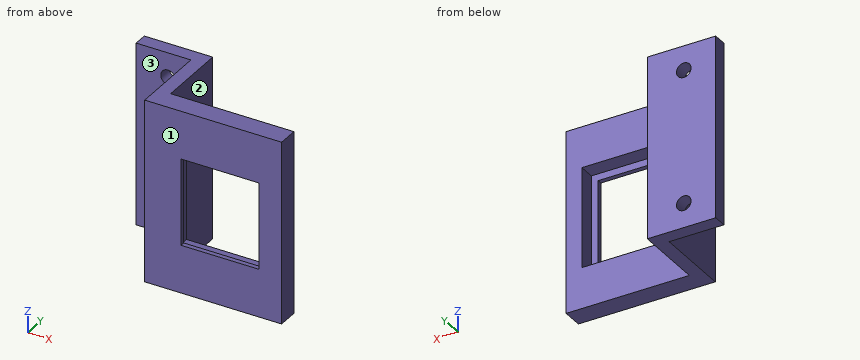
from build123d import *

# Parameters (mm, degrees)
BOSS_EXTRUDE1_DEPTH = 40
SKETCH2_W           = 20.1
SKETCH2_H           = 22
CUT_EXTRUDE1_DEPTH  = 3.5
SKETCH3_W           = 17.1
SKETCH3_H           = 19
CUT_EXTRUDE2_DEPTH  = 54.488316481
SKETCH4_R           = 1.6
CUT_EXTRUDE3_DEPTH  = 54.851648071


with BuildPart() as part:
    # Sketch1 → Boss-Extrude1 (new body)
    with BuildSketch(Plane.XY):
        Polygon((0, 0), (0, 17), (-12, 17), (-12, 20), (3, 20), (3, 4.5), (30, 4.5), (30, 0), align=None)
    extrude(amount=-BOSS_EXTRUDE1_DEPTH)

    # Sketch2 → Cut-Extrude1 (cut)
    with BuildSketch(Plane(origin=(0, 4.5, 0), x_dir=(1, 0, 0), z_dir=(0, 1, 0))):
        with Locations((16.5, 20)):
            Rectangle(SKETCH2_W, SKETCH2_H)
    extrude(amount=-CUT_EXTRUDE1_DEPTH, mode=Mode.SUBTRACT)

    # Sketch3 → Cut-Extrude2 (cut, through all)
    with BuildSketch(Plane(origin=(0, 1, 0), x_dir=(1, 0, 0), z_dir=(0, 1, 0))):
        with Locations((16.5, 20)):
            Rectangle(SKETCH3_W, SKETCH3_H)
    extrude(amount=-CUT_EXTRUDE2_DEPTH, mode=Mode.SUBTRACT)

    # Sketch4 → Cut-Extrude3 (cut, through all)
    with BuildSketch(Plane(origin=(0, 20, 0), x_dir=(1, 0, 0), z_dir=(0, 1, 0))):
        with Locations(Location((-5, 34.63, 0), (0, 0, 270))):
            Circle(SKETCH4_R)
        with Locations(Location((-5, 5.366, 0), (0, 0, 270))):
            Circle(SKETCH4_R)
    extrude(amount=-CUT_EXTRUDE3_DEPTH, mode=Mode.SUBTRACT)


solid = part.part
For this review, take the finished solid that the model builds, in its own axes (mm). Face numbers are marked on the shaded views. A direction names the side the tool comes from. Round coordinates to 2 decimals unless told otherwise and drop trailing zeros. Order: outer loops, then holes, each group sorted by start corner. A loop starts at its lowest first (then second) coordinate and runs counter-clockwise, first axis right, second up. Notation, with made-up numbers: M 15.25,82 L 60.25,82 A18 ccw 60.25,86 Z; hole C 55,-2.75 d3. An arc over 180 degrees is marked long. Use a Markdown table: item, result. Add a question column.
Item 1: Insertion check: pin 1 (0.5 mm diameter, centred on y = 0.5, z = -23, fed in from -X); pin 2 (1.5 mm diameter, centred on x = 10, z = -15, fed in from -Y); pin 3 (1.5 mm diameter, centred on y = 8.5, z = -22.5, fed in from +X); pin 4 (16 mm diameter, centred on x = 19.5, z = -15.5, fed in from +Y). Each pin has a flat end and moves straight along its axis. Give the tip position at first contact, or say it passes through.
Item 2: Add section D-D, the plane z = -34.63. Give the boundary of the cut face in (x, y), then the cut area to 3 significant figures.
Item 3: Add section A-A, the plane x = 9. Give the boundary of the cut face in (y, z).
Item 4: To check wall thickness, follow line 1 along X through (y, z) = (18.85, -34.63); line 2 along X through (y, z) = (2, -27.5); line 3 along Z through (x, y) = (16, 3.5). State the ranges of each line that lie inside material, in increasing order.
Item 5: Add section B-B, the plane z = -28. Give the boundary of the cut face in (x, y).
Item 6: Tool access review of the marked faces 1, 2 and 3: name each direction out of +Z, -Z, +X, -X, +Y, -Y from which nothing blocks a thin tool from reaching the whole face with its end or side.
Item 7: Add section C-C, the plane x = -5. Give the boundary of the cut face in (y, z).
Geometry results:
| question | item | result |
|---|---|---|
| 1 | pin 1 | stops at x = 0 |
| 1 | pin 2 | passes through |
| 1 | pin 3 | stops at x = 3 |
| 1 | pin 4 | stops at y = 4.5 |
| 2 | outline | M -12,17 L -6.6,17 L -6.6,20 L -12,20 Z; M -3.4,17 L 0,17 L 0,0 L 30,0 L 30,4.5 L 3,4.5 L 3,20 L -3.4,20 Z |
| 2 | area | 208 mm² |
| 3 | outline | M 0,-40 L 4.5,-40 L 4.5,-31 L 1,-31 L 1,-29.5 L 0,-29.5 Z; M 0,-10.5 L 1,-10.5 L 1,-9 L 4.5,-9 L 4.5,0 L 0,0 Z |
| 4 | line 1 | x = -12 to -6.6, -3.4 to 3 |
| 4 | line 2 | x = 0 to 6.45, 26.55 to 30 |
| 4 | line 3 | z = -40 to -31, -9 to 0 |
| 5 | outline | M -12,17 L 0,17 L 0,0 L 7.95,0 L 7.95,1 L 6.45,1 L 6.45,4.5 L 3,4.5 L 3,20 L -12,20 Z; M 25.05,0 L 30,0 L 30,4.5 L 26.55,4.5 L 26.55,1 L 25.05,1 Z |
| 6 | face 1 | +Z, -Z, +X, -X, -Y |
| 6 | face 2 | +Z, -Z, +X, +Y |
| 6 | face 3 | +Z, -Z, -X, -Y |
| 7 | outline | M 17,-40 L 20,-40 L 20,-36.23 L 17,-36.23 Z; M 17,-33.03 L 20,-33.03 L 20,-6.97 L 17,-6.97 Z; M 17,-3.77 L 20,-3.77 L 20,0 L 17,0 Z |
